from build123d import *

# Parameters (mm, degrees)
SKETCH2_W               = 95
SKETCH2_H               = 50
BOSS_EXTRUDE1_DEPTH     = 3
SKETCH1_R               = 2
SKETCH1_R_2             = 1.5
CUT_EXTRUDE2_DEPTH      = 4
CUT_EXTRUDE2_DEPTH_BACK = 1


with BuildPart() as part:
    # Sketch2 → Boss-Extrude1 (new body)
    with BuildSketch(Plane.XY):
        Rectangle(SKETCH2_W, SKETCH2_H)
    extrude(amount=BOSS_EXTRUDE1_DEPTH)

    # Sketch1 → Cut-Extrude2 (cut, two sides)
    with BuildSketch(Plane.XY) as cut_extrude2_sk:
        with BuildLine():
            ThreePointArc((18.25, -5.629165125), (19.596194078, -4.596194078), (20.629165125, -3.25))
            Line((20.629165125, -3.25), (29.370834875, -3.25))
            ThreePointArc((29.370834875, -3.25), (35, -6.5), (40.629165125, -3.25))
            Line((40.629165125, -3.25), (41, -3.25))
            Line((41, -3.25), (41, -13.147782503))
            ThreePointArc((41, -13.147782503), (37.464466094, -14.964466094), (35.647782503, -18.5))
            Line((35.647782503, -18.5), (18.25, -18.5))
            Line((18.25, -18.5), (18.25, -5.629165125))
        make_face()
        with BuildLine():
            ThreePointArc((40.629165125, 3.25), (35, 6.5), (29.370834875, 3.25))
            Line((29.370834875, 3.25), (20.629165125, 3.25))
            ThreePointArc((20.629165125, 3.25), (19.596194078, 4.596194078), (18.25, 5.629165125))
            Line((18.25, 5.629165125), (18.25, 18.5))
            Line((18.25, 18.5), (35.647782503, 18.5))
            ThreePointArc((35.647782503, 18.5), (37.464466094, 14.964466094), (41, 13.147782503))
            Line((41, 13.147782503), (41, 3.25))
            Line((41, 3.25), (40.629165125, 3.25))
        make_face()
        with BuildLine():
            ThreePointArc((11.75, 5.629165125), (10.403805922, 4.596194078), (9.370834875, 3.25))
            Line((9.370834875, 3.25), (-9.370834875, 3.25))
            ThreePointArc((-9.370834875, 3.25), (-10.403805922, 4.596194078), (-11.75, 5.629165125))
            Line((-11.75, 5.629165125), (-11.75, 18.5))
            Line((-11.75, 18.5), (11.75, 18.5))
            Line((11.75, 18.5), (11.75, 5.629165125))
        make_face()
        with BuildLine():
            ThreePointArc((-11.75, -5.629165125), (-10.403805922, -4.596194078), (-9.370834875, -3.25))
            Line((-9.370834875, -3.25), (9.370834875, -3.25))
            ThreePointArc((9.370834875, -3.25), (10.403805922, -4.596194078), (11.75, -5.629165125))
            Line((11.75, -5.629165125), (11.75, -18.5))
            Line((11.75, -18.5), (-11.75, -18.5))
            Line((-11.75, -18.5), (-11.75, -5.629165125))
        make_face()
        with Locations((-15, 0)):
            Circle(SKETCH1_R)
        with BuildLine():
            ThreePointArc((-18.25, 5.629165125), (-19.596194078, 4.596194078), (-20.629165125, 3.25))
            Line((-20.629165125, 3.25), (-41, 3.25))
            Line((-41, 3.25), (-41, 13.147782503))
            ThreePointArc((-41, 13.147782503), (-37.464466094, 14.964466094), (-35.647782503, 18.5))
            Line((-35.647782503, 18.5), (-18.25, 18.5))
            Line((-18.25, 18.5), (-18.25, 5.629165125))
        make_face()
        with BuildLine():
            ThreePointArc((-20.629165125, -3.25), (-19.596194078, -4.596194078), (-18.25, -5.629165125))
            Line((-18.25, -5.629165125), (-18.25, -18.5))
            Line((-18.25, -18.5), (-35.647782503, -18.5))
            ThreePointArc((-35.647782503, -18.5), (-37.464466094, -14.964466094), (-41, -13.147782503))
            Line((-41, -13.147782503), (-41, -3.25))
            Line((-41, -3.25), (-20.629165125, -3.25))
        make_face()
        with Locations((42.060660172, -19.560660172)):
            Circle(SKETCH1_R_2)
        with Locations((42.060660172, 19.560660172)):
            Circle(SKETCH1_R_2)
        with Locations((15, 0)):
            Circle(SKETCH1_R)
        with Locations((35, 0)):
            Circle(SKETCH1_R)
        with Locations((-42.060660172, 19.560660172)):
            Circle(SKETCH1_R_2)
        with Locations((-42.060660172, -19.560660172)):
            Circle(SKETCH1_R_2)
    extrude(amount=CUT_EXTRUDE2_DEPTH, mode=Mode.SUBTRACT)
    extrude(cut_extrude2_sk.sketch, amount=-CUT_EXTRUDE2_DEPTH_BACK, mode=Mode.SUBTRACT)


solid = part.part
Source: CAD feature listing. Evaluate the final solid. Frame: model axes, mm. A direction names the side the tool comes from. Coordinates: 2 decimals unless noted, no trailing zeros. Loops run counter-clockwise (first coordinate to the right, second up) from the corner with the lowest first, then second, coordinate; pieces in that order, holes last. Notation, with made-up numbers: (70.25, 42.5) - (108.25, 42.5) arc R25 cw to (108.25, 81.5) - close; hole circle Ø3 at (-13, 68.5). An arc over 180 degrees is marked (long way). One line per question, with ' | ' between items.
1) Pull-direction query (Y, two-part tool) for faces 3 (the face through (-1, -25, 1)), 4 (the face through (-37.505, 14.925, 1.479)), 5 (the face through (-1, 0, 0)); classes: released by +Y, released by -Y, zero draft, split by the parting line, or undercut.
Report:
face 3: released by -Y | face 4: undercut | face 5: zero draft
2) Section A-A, the plane y = 0. Return loops of the section in (x, z).
Report:
outline: (-47.5, 0) - (-17, 0) - (-17, 3) - (-47.5, 3) - close; (-13, 0) - (13, 0) - (13, 3) - (-13, 3) - close; (17, 0) - (33, 0) - (33, 3) - (17, 3) - close; (37, 0) - (47.5, 0) - (47.5, 3) - (37, 3) - close
3) Section C-C, the plane x = -39.5. Return loops of the section in (y, z), then the cut area to 3 significant figures.
Report:
outline: (-25, 0) - (-13.59, 0) - (-13.59, 3) - (-25, 3) - close; (-3.25, 0) - (3.25, 0) - (3.25, 3) - (-3.25, 3) - close; (13.59, 0) - (25, 0) - (25, 3) - (13.59, 3) - close | area: 88.0 mm²
4) Section B-B, the plane x = -15. Return loops of the section in (y, z).
Report:
outline: (-25, 0) - (-2, 0) - (-2, 3) - (-25, 3) - close; (2, 0) - (25, 0) - (25, 3) - (2, 3) - close
5) Line query: line 1 along X through (y, z) = (0, 1.75); line 2 along Y through (x, z) = (-7, 1.35); line 3 along X through (y, z) = (-12.5, 2.65). Output: solid intervals per line, ascending.
Report:
line 1: x = -47.5 to -17, -13 to 13, 17 to 33, 37 to 47.5 | line 2: y = -25 to -18.5, -3.25 to 3.25, 18.5 to 25 | line 3: x = -47.5 to -41, -18.25 to -11.75, 11.75 to 18.25, 41 to 47.5
6) First-contact query: P1, Ø1.5, axis at x = -8, y = -17, coming from the -Z side. Flat tip, straight axial feed; report the tip coordinate or a pass-through.
Report:
P1: passes through
7) Section D-D, the plane y = 8.5. Return loops of the section in (x, z).
Report:
outline: (-47.5, 0) - (-41, 0) - (-41, 3) - (-47.5, 3) - close; (-18.25, 0) - (-11.75, 0) - (-11.75, 3) - (-18.25, 3) - close; (11.75, 0) - (18.25, 0) - (18.25, 3) - (11.75, 3) - close; (41, 0) - (47.5, 0) - (47.5, 3) - (41, 3) - close
8) Set-up query: faces 1 (the face through (-1, 0, 3)), 2 (the face through (-19.58, 4.61, 1.48)). Return all of +Z, -Z, +X, -X, +Y, -Y with unobstructed straight access to the full face (end or side cutting, diameter ignored); none if empty.
Report:
face 1: +Z, +X, -X, +Y, -Y | face 2: +Z, -Z
